Can you work these out from the drawing? Everything is in mm from the part's minimum corner. A direction names the side the tool comes from. Give positions to 0.01 mm unless a question says otherwise; leave off trailing zeros. Write each loop counter-clockwise with the first axis right and the second up, starting at its lowest first coordinate (ties: lowest second). Pieces come first, ordered by that corner, then holes. Notation, with made-up numbers: M 51,71 L 62,71 A22 cw 62,104 Z; hole C 69,1 d7. An arc over 180 degrees is marked long. One line per item, written item: value.
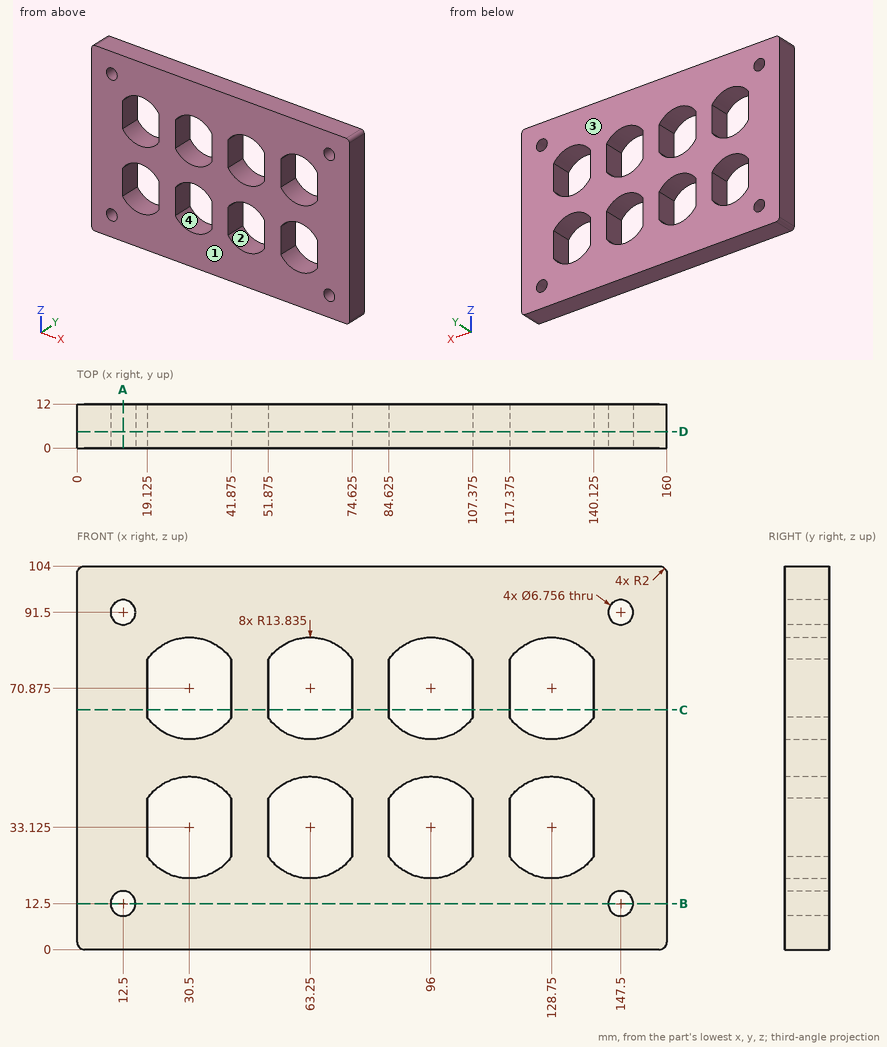
1) If we section it at C-C, the plane z = 65: Write out the boundary of the cut face in (x, y) (3 decimals), then the cut area to 3 significant figures.
Outcome:
outline: M 0,0 L 19.125,0 L 19.125,12 L 0,12 Z; M 41.875,0 L 51.875,0 L 51.875,12 L 41.875,12 Z; M 74.625,0 L 84.625,0 L 84.625,12 L 74.625,12 Z; M 107.375,0 L 117.375,0 L 117.375,12 L 107.375,12 Z; M 140.125,0 L 160,0 L 160,12 L 140.125,12 Z
area: 828 mm^2
2) I'm going to push a flat-ended pin straight in: pin 1 (3.5 mm diameter, centred on y = 3.5, z = 67.5, fed in from -X). Where does the tip first touch, or does it pass through?
Outcome:
pin 1: stops at x = 0
3) If we section it at D-D, the plane y = 4.5: Give the number of separate pieces and of enclosed holes in the cut face, then the cut area to 3 significant figures.
Outcome:
separate pieces: 1
enclosed holes: 12
area: 12,100 mm^2
4) On a 3-axis mill with a long thin cutter (end or side, diameter ignored), from which of +Z, -Z, +X, -X, +Y, -Y can I reach the whole of each face in a straight line? I mean the marked faces 1 and 2. Say none if no direction works.
Outcome:
face 1: +Z, -Z, +X, -X, -Y
face 2: +Y, -Y
5) If we section it at B-B, the plane z = 12.5: Write out the boundary of the cut face in (x, y), then the cut area to 3 significant figures.
Outcome:
outline: M 0,0 L 9.12,0 L 9.12,12 L 0,12 Z; M 15.88,0 L 144.12,0 L 144.12,12 L 15.88,12 Z; M 150.88,0 L 160,0 L 160,12 L 150.88,12 Z
area: 1,760 mm^2
6) If we section it at A-A, the plane x = 12.5: Write out the boundary of the cut face in (y, z), then the cut area to 3 significant figures.
Outcome:
outline: M 0,0 L 12,0 L 12,9.12 L 0,9.12 Z; M 0,15.88 L 12,15.88 L 12,88.12 L 0,88.12 Z; M 0,94.88 L 12,94.88 L 12,104 L 0,104 Z
area: 1,090 mm^2
7) We'd pull the mould along Z, two halves only. Please class the marked faces 3 and 4: pulls with the +Z half, pulls with the -Z half, needs draft (parallel to the pull), parting line crosses it, or undercut.
Outcome:
face 3: needs draft
face 4: undercut
8) Please list where these lines run through material, in increasing order: L1, parallel to X at y = 4, z = 12.5; L2, parallel to X at y = 6.75, z = 38 (3 decimals); L3, parallel to Z at x = 147.5, y = 6.75. Write a range as from..to.
Outcome:
L1: x = 0..9.12, 15.88..144.12, 150.88..160
L2: x = 0..19.125, 41.875..51.875, 74.625..84.625, 107.375..117.375, 140.125..160
L3: z = 0..9.12, 15.88..88.12, 94.88..104
